Read the model definition and answer for the solid it produces. Units are mm, in the model's axes. Face numbers are marked on the shaded views. Coordinates: 2 decimals unless noted, no trailing zeros. Write each loop counter-clockwise with the first axis right and the second up, starting at its lowest first coordinate (ties: lowest second). Pieces come first, ordered by that corner, then holes. Notation, with made-up numbers: (-22.75, 53.5) - (-11.75, 53.5) arc R18 cw to (-11.75, 83.5) - close; hole circle Ø11 at (32, 75.25). An arc over 180 degrees is marked (long way). Return JSON: item names as keys, results as strings.
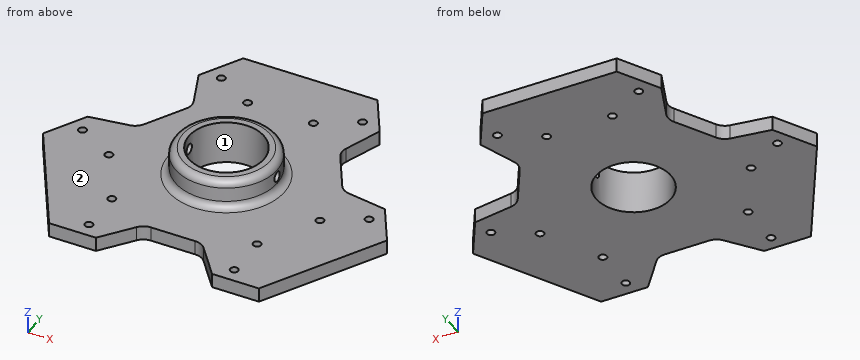
```python
from build123d import *

# Parameters (mm, degrees)
SKETCH011_R        = 25.8
PAD007_DEPTH       = 10
SKETCH012_R        = 2.75
POCKET003_DEPTH    = 636.6056068561
POLARPATTERN_COUNT = 3
SKETCH_R           = 35
SKETCH_R_2         = 25.8
PAD_DEPTH          = 20
FILLET_R           = 5
SKETCH013_R        = 3.5
POCKET_DEPTH       = 118.3578051839
POCKET_DEPTH_BACK  = 118.3578051839
FILLET001_R        = 10


with BuildPart() as part:
    # Sketch011 → Pad007 (new body)
    with BuildSketch(Plane.XY):
        Polygon((-46.1880215352, 110), (46.1880215352, 110), (118.3568051839, -15), (72.1687836487, -95), (-72.1687836487, -95), (-118.3568051839, -15), align=None)
        Circle(SKETCH011_R, mode=Mode.SUBTRACT)
    extrude(amount=PAD007_DEPTH)

    # Sketch012 → Pocket003 (cut, through all)
    with BuildSketch(Plane.XY):
        with Locations((-48.6121593217, 85.8012701892)):
            Circle(SKETCH012_R)
        with Locations((-98.6121593217, -0.8012701892)):
            Circle(SKETCH012_R)
        with Locations((-22.6313972081, 70.8012701892)):
            Circle(SKETCH012_R)
        with Locations((-72.6313972081, -15.8012701892)):
            Circle(SKETCH012_R)
        Polygon((-62.2724133595, 82.1410161514), (-50.6217782649, 52.3205080757), (-70.6217782649, 17.6794919243), (-102.2724133595, 12.8589838486), align=None)
    pocket003 = extrude(amount=POCKET003_DEPTH, mode=Mode.SUBTRACT)

    # PolarPattern: Pocket003 ×3 about axis
    polarpattern_axis = Axis((0, 0, 0), (0, 0, 1))
    for i in range(1, POLARPATTERN_COUNT):
        add(pocket003.rotate(polarpattern_axis, i * 360 / POLARPATTERN_COUNT), mode=Mode.SUBTRACT)

    # Sketch (on Face5 of PolarPattern) → Pad (join)
    with BuildSketch(Plane.XY.offset(10)):
        Circle(SKETCH_R)
        Circle(SKETCH_R_2, mode=Mode.SUBTRACT)
    extrude(amount=PAD_DEPTH)

    # Fillet
    fillet_edges = [part.edges().sort_by_distance(p)[0] for p in [
        (-35, 0, 10),
        (-35, 0, 30),
    ]]
    fillet(fillet_edges, radius=FILLET_R)

    # Sketch013 (on DatumPlane) → Pocket (cut, two sides)
    with BuildSketch(Plane(origin=(0, 0, 15), x_dir=(0, 0, -1), z_dir=(1, 0, 0))) as pocket_sk:
        with Locations((-5, 0)):
            Circle(SKETCH013_R)
    extrude(amount=-POCKET_DEPTH, mode=Mode.SUBTRACT)
    extrude(pocket_sk.sketch, amount=POCKET_DEPTH_BACK, mode=Mode.SUBTRACT)

    # Fillet001
    fillet001_edges = [part.edges().sort_by_distance(p)[0] for p in [
        (20, -70, 5),
        (-20, -70, 5),
        (50.621778, 52.320508, 5),
        (70.621778, 17.679492, 5),
        (-50.621778, 52.320508, 5),
        (-70.621778, 17.679492, 5),
    ]]
    fillet(fillet001_edges, radius=FILLET001_R)


solid = part.part
```
(1) Straight lines are drawn through the part: line 1 (X direction, y = -0.5, z = 7); line 2 (X direction, y = -18, z = 9); line 3 (Z direction, x = 41.5, y = -6.5). For each, find the intervals that lie inside material, in ascending order. Write a range as from..to.
Answer:
{"line 1": "-109.99..-101.35, -95.88..-25.8, 25.8..95.88, 101.35..109.99", "line 2": "-116.62..-74.28, -70.98..-18.48, 18.48..70.98, 74.28..116.62", "line 3": "0..10"}
(2) Flat-ended cylindrical pins translate along their axes: P1, Ø11, axis at x = -7.5, z = 6.5, coming from the -Y side; P2, Ø4.5, axis at x = -50, y = -55, coming from the +Z side; P3, Ø4, axis at x = 23, y = -61.5, coming from the +Z side; P4, Ø1, axis at x = -4, z = 19.5, coming from the -Y side. Find the tip coordinate at first contact, or state that the pin passes through.
Answer:
{"P1": "y = -70", "P2": "through", "P3": "z = 10", "P4": "y = -34.82"}
(3) Determine the mould class of the marked faces 1 and 2 for opening direction Y: +Y half, -Y half, draft (parallel to the pull), parting line (faces both ways), or undercut.
Answer:
{"face 1": "undercut", "face 2": "draft"}
(4) A cutting plane is placed at C-C (z = 7). State how many separate pieces and enclosed holes the cut face has, and give its area (3 significant figures).
Answer:
{"separate pieces": "1", "enclosed holes": "13", "area": "29,000 mm²"}
(5) A cutting plane is placed at A-A (x = 0). Determine the outline of the cut face in (y, z), and give its area (3 significant figures).
Answer:
{"outline": "(-70, 0) - (-25.8, 0) - (-25.8, 30) - (-30, 30) arc R5 ccw to (-35, 25) - (-35, 15) arc R5 cw to (-40, 10) - (-70, 10) - close; (25.8, 0) - (110, 0) - (110, 10) - (40, 10) arc R5 cw to (35, 15) - (35, 25) arc R5 ccw to (30, 30) - (25.8, 30) - close", "area": "1,650 mm²"}
(6) A cutting plane is placed at D-D (y = 97). Determine the outline of the cut face in (x, z).
Answer:
{"outline": "(-53.69, 0) - (53.69, 0) - (53.69, 10) - (-53.69, 10) - close"}
(7) A cutting plane is placed at B-B (y = -77). Determine the outline of the cut face in (x, z), and give its area (3 significant figures).
Answer:
{"outline": "(-82.56, 0) - (-25.6, 0) - (-25.6, 10) - (-82.56, 10) - close; (25.6, 0) - (82.56, 0) - (82.56, 10) - (25.6, 10) - close", "area": "1,140 mm²"}
